from build123d import *

# Parameters (mm, degrees)
SKETCH1_W           = 26.5
SKETCH1_H           = 19.2
BOSS_EXTRUDE1_DEPTH = 1.5
SKETCH2_W           = 12.5
SKETCH2_H           = 3.5
BOSS_EXTRUDE2_DEPTH = 3.5
CUT_EXTRUDE1_DEPTH  = 18
SKETCH4_W           = 12.5
SKETCH4_H           = 0.5
BOSS_EXTRUDE3_DEPTH = 5
BOSS_EXTRUDE4_DEPTH = 0.5


with BuildPart() as part:
    # Sketch1 → Boss-Extrude1 (new body)
    with BuildSketch(Plane(origin=(0, 0, 0), x_dir=(1, 0, 0), z_dir=(0, 1, 0))):
        with Locations((3.967391304, -3.07826087)):
            Rectangle(SKETCH1_W, SKETCH1_H)
    extrude(amount=BOSS_EXTRUDE1_DEPTH)

    # Sketch2 → Boss-Extrude2 (add)
    with BuildSketch(Plane.XY.offset(12.67826087)):
        with Locations((3.967391304, 1.76)):
            Rectangle(SKETCH2_W, SKETCH2_H)
    extrude(amount=BOSS_EXTRUDE2_DEPTH)

    # Sketch3 → Cut-Extrude1 (cut)
    with BuildSketch(Plane.ZY.offset(2.282608696)):
        with BuildLine():
            Line((14.17826087, 3.01), (12.67826087, 3.01))
            Line((12.67826087, 3.01), (12.67826087, 1.5))
            Line((12.67826087, 1.5), (12.67826087, 0.336807219))
            Line((12.67826087, 0.336807219), (14.17826087, 0.336807219))
            ThreePointArc((14.17826087, 0.336807219), (15.439541787, 1.67340361), (14.17826087, 3.01))
        make_face()
        with BuildLine():
            Line((16.17826087, 3.51), (14.17826087, 3.51))
            ThreePointArc((14.17826087, 3.51), (15.93151881, 1.860671544), (14.392294136, 0.01))
            Line((14.392294136, 0.01), (16.17826087, 0.01))
            Line((16.17826087, 0.01), (16.17826087, 3.51))
        make_face()
    extrude(amount=-CUT_EXTRUDE1_DEPTH, mode=Mode.SUBTRACT)

    # Sketch4 → Boss-Extrude3 (add)
    with BuildSketch(Plane(origin=(0, 0, 12.67826087), x_dir=(-1, 0, 0), z_dir=(0, 0, -1))):
        with Locations((-3.967391304, 3.26)):
            Rectangle(SKETCH4_W, SKETCH4_H)
    extrude(amount=BOSS_EXTRUDE3_DEPTH)

    # Sketch6 → Boss-Extrude4 (add)
    with BuildSketch(Plane(origin=(0, 3.51, 0), x_dir=(1, 0, 0), z_dir=(0, 1, 0))):
        Polygon((-2.282608696, -7.67826087), (-6.782608696, -7.67826087), (-2.282608696, -12.67826087), align=None)
        Polygon((10.217391304, -7.67826087), (14.717391304, -7.67826087), (10.217391304, -12.67826087), align=None)
    extrude(amount=-BOSS_EXTRUDE4_DEPTH)


solid = part.part
Design review of the part built by this model. Coordinates are the model's own, in mm. A direction names the side the tool comes from. Give positions to 0.01 mm unless a question says otherwise; leave off trailing zeros. Order: outer loops, then holes, each group sorted by start corner. A loop starts at its lowest first (then second) coordinate and runs counter-clockwise, first axis right, second up. Notation, with made-up numbers: (40, 48.5) - (61, 48.5) arc R16 ccw to (61, 67.5) - close; hole circle Ø11 at (-3.75, -18). An arc over 180 degrees is marked (long way). Use CSV: the item, a comma, the result in double quotes. Start each with the question number.
Q1. For line 1 (Y direction, x = 8, z = 8.75); line 2 (Y direction, x = -6.25, z = -2.5); line 3 (Y direction, x = 7, z = 13.25), list the stretches that pass through material, from the lowest coordinate up.
Q2. Machinability: for faces 4 (the face through (4, 0.337, 13)), 5 (the face through (-4.564, 3.263, 10.143)), 6 (the face through (12.5, 3.26, 10.14)), which of the approach directions +Z, -Z, +X, -X, +Y, -Y give a long, thin tool a straight path to every point of the face, cutting with its end or side? Answer none if there is none.
Q3. For P1, Ø2, axis at x = -4.5, z = 3, coming from the +Y side; P2, Ø0.8, axis at x = 5.5, y = 1, coming from the +Z side; P3, Ø1.4, axis at x = 4.5, z = 13.5, coming from the -Y side, all flat-tipped, find the tip position at first contact; note any pin that passes through.
Q4. Draft analysis for pull direction Y (two halves, no side actions). For faces 1 (the face through (-2.283, 3, 15)), 2 (the face through (4, 0.01, 14)), 3 (the face through (4, 1.5, 3)), state which applies: pulls with the +Y half, pulls with the -Y half, needs draft (parallel to the pull), parting line crosses it, or undercut.
Q5. Take a section at D-D (z = 6.25). State the section outline as (x, y) points, and give its area (4 significant figures).
Q6. Take a section at C-C (y = 0.9). State the section outline as (x, z) points.
Q7. Take a section at A-A (z = 13.5). State the section outline as (x, y) points, and give its area (3 significant figures).
Calculated:
1,line 1,"y = 0 to 1.5, 3.01 to 3.51"
1,line 2,"y = 0 to 1.5"
1,line 3,"y = 0.01 to 0.34, 3.01 to 3.51"
2,face 4,"+X, -X"
2,face 5,"+Z, -X, +Y"
2,face 6,"+Z, +X, +Y"
3,P1,"stops at y = 1.5"
3,P2,"stops at z = 15.9"
3,P3,"stops at y = 0.01"
4,face 1,"needs draft"
4,face 2,"pulls with the -Y half"
4,face 3,"undercut"
5,outline,"(-9.28, 0) - (17.22, 0) - (17.22, 1.5) - (-9.28, 1.5) - close"
5,area,"39.75 mm²"
6,outline,"(-9.28, -6.52) - (17.22, -6.52) - (17.22, 12.68) - (-9.28, 12.68) - close; (-2.28, 15.19) - (10.22, 15.19) - (10.22, 15.71) - (-2.28, 15.71) - close"
7,outline,"(-2.28, 0.01) - (10.22, 0.01) - (10.22, 0.34) - (-2.28, 0.34) - close; (-2.28, 3.01) - (10.22, 3.01) - (10.22, 3.51) - (-2.28, 3.51) - close"
7,area,"10.3 mm²"
